Verification items for the finished model (mm, model axes). Coordinates: 2 decimals unless noted, no trailing zeros. Write each loop counter-clockwise with the first axis right and the second up, starting at its lowest first coordinate (ties: lowest second). Pieces come first, ordered by that corner, then holes. Notation, with made-up numbers: (32, 44) -> (61, 44) arc R25 cw to (61, 76) -> close; hole circle Ø11 at (26.25, 60.5). An arc over 180 degrees is marked (long way). Use a Markdown table: item, result. Add a question column.
from build123d import *

# Parameters (mm, degrees)
F1_DEPTH = 10.16


with BuildPart() as f1:
    # F0 (on Top) → F1 (new body)
    with BuildSketch(Plane.XY):
        with BuildLine():
            Line((-127, 50.8), (-127, 0))
            Line((-127, 0), (-115.57, 0))
            ThreePointArc((-115.57, 0), (-107.95, 7.62), (-100.33, 0))
            Line((-100.33, 0), (-88.9, 0))
            ThreePointArc((-88.9, 0), (-81.572297, 35.343604), (-60.79718, 64.860719))
            Line((-60.79718, 64.860719), (-77.096278, 79.650577))
            ThreePointArc((-77.096278, 79.650577), (-87.859909, 79.128047), (-88.382439, 89.891679))
            Line((-88.382439, 89.891679), (-104.681537, 104.681537))
            ThreePointArc((-104.681537, 104.681537), (-121.19962, 79.960478), (-127, 50.8))
        make_face()
        with BuildLine():
            ThreePointArc((-50.8, 127), (-79.960478, 121.19962), (-104.681537, 104.681537))
            Line((-104.681537, 104.681537), (-88.382439, 89.891679))
            ThreePointArc((-88.382439, 89.891679), (-79.994898, 91.879738), (-75.119358, 84.771128))
            ThreePointArc((-75.119358, 84.771128), (-75.630748, 82.026668), (-77.096278, 79.650577))
            Line((-77.096278, 79.650577), (-60.79718, 64.860719))
            ThreePointArc((-60.79718, 64.860719), (-32.688622, 82.672027), (0, 88.9))
            Line((0, 88.9), (0, 100.33))
            ThreePointArc((0, 100.33), (-7.62, 107.95), (0, 115.57))
            Line((0, 115.57), (0, 127))
            Line((0, 127), (-50.8, 127))
        make_face()
        with BuildLine():
            Line((89.270123, 89.048531), (104.681537, 104.681537))
            ThreePointArc((104.681537, 104.681537), (79.960478, 121.19962), (50.8, 127))
            Line((50.8, 127), (0, 127))
            Line((0, 127), (0, 115.57))
            ThreePointArc((0, 115.57), (5.388154, 113.338154), (7.62, 107.95))
            ThreePointArc((7.62, 107.95), (5.388154, 102.561846), (0, 100.33))
            Line((0, 100.33), (0, 88.9))
            ThreePointArc((0, 88.9), (34.215472, 82.051883), (63.159593, 62.562575))
            Line((63.159593, 62.562575), (78.571008, 78.19558))
            ThreePointArc((78.571008, 78.19558), (78.49409, 88.971613), (89.270123, 89.048531))
        make_face()
        with BuildLine():
            Line((115.57, 0), (127, 0))
            Line((127, 0), (127, 50.8))
            ThreePointArc((127, 50.8), (121.19962, 79.960478), (104.681537, 104.681537))
            Line((104.681537, 104.681537), (89.270123, 89.048531))
            ThreePointArc((89.270123, 89.048531), (90.950075, 86.56321), (91.540565, 83.622056))
            ThreePointArc((91.540565, 83.622056), (86.861719, 76.592545), (78.571008, 78.19558))
            Line((78.571008, 78.19558), (63.159593, 62.562575))
            ThreePointArc((63.159593, 62.562575), (82.213435, 33.82545), (88.9, 0))
            Line((88.9, 0), (100.33, 0))
            ThreePointArc((100.33, 0), (107.95, 7.62), (115.57, 0))
        make_face()
        with BuildLine():
            Line((88.958455, -89.357986), (104.681537, -104.681537))
            ThreePointArc((104.681537, -104.681537), (121.19962, -79.960478), (127, -50.8))
            Line((127, -50.8), (127, 0))
            Line((127, 0), (115.57, 0))
            ThreePointArc((115.57, 0), (107.95, -7.62), (100.33, 0))
            Line((100.33, 0), (88.9, 0))
            ThreePointArc((88.9, 0), (81.986502, -34.371843), (62.321292, -63.397685))
            Line((62.321292, -63.397685), (78.044374, -78.721236))
            ThreePointArc((78.044374, -78.721236), (86.372107, -76.981033), (91.121415, -84.039611))
            ThreePointArc((91.121415, -84.039611), (90.559993, -86.910304), (88.958455, -89.357986))
        make_face()
        with BuildLine():
            Line((0, -115.57), (0, -127))
            Line((0, -127), (50.8, -127))
            ThreePointArc((50.8, -127), (79.960478, -121.19962), (104.681537, -104.681537))
            Line((104.681537, -104.681537), (88.958455, -89.357986))
            ThreePointArc((88.958455, -89.357986), (78.18304, -89.496652), (78.044374, -78.721236))
            Line((78.044374, -78.721236), (62.321292, -63.397685))
            ThreePointArc((62.321292, -63.397685), (33.668648, -82.277774), (0, -88.9))
            Line((0, -88.9), (0, -100.33))
            ThreePointArc((0, -100.33), (5.388154, -102.561846), (7.62, -107.95))
            ThreePointArc((7.62, -107.95), (5.388154, -113.338154), (0, -115.57))
        make_face()
        with BuildLine():
            ThreePointArc((-104.681537, -104.681537), (-79.960478, -121.19962), (-50.8, -127))
            Line((-50.8, -127), (0, -127))
            Line((0, -127), (0, -115.57))
            ThreePointArc((0, -115.57), (-7.62, -107.95), (0, -100.33))
            Line((0, -100.33), (0, -88.9))
            ThreePointArc((0, -88.9), (-34.133071, -82.086195), (-63.033834, -62.689279))
            Line((-63.033834, -62.689279), (-78.491774, -78.275104))
            ThreePointArc((-78.491774, -78.275104), (-76.823745, -80.754866), (-76.237686, -83.685408))
            ThreePointArc((-76.237686, -83.685408), (-80.927144, -90.719349), (-89.223597, -89.095712))
            Line((-89.223597, -89.095712), (-104.681537, -104.681537))
        make_face()
        with BuildLine():
            ThreePointArc((-127, -50.8), (-121.19962, -79.960478), (-104.681537, -104.681537))
            Line((-104.681537, -104.681537), (-89.223597, -89.095712))
            ThreePointArc((-89.223597, -89.095712), (-89.26799, -78.319496), (-78.491774, -78.275104))
            Line((-78.491774, -78.275104), (-63.033834, -62.689279))
            ThreePointArc((-63.033834, -62.689279), (-82.179431, -33.907979), (-88.9, 0))
            Line((-88.9, 0), (-100.33, 0))
            ThreePointArc((-100.33, 0), (-107.95, -7.62), (-115.57, 0))
            Line((-115.57, 0), (-127, 0))
            Line((-127, 0), (-127, -50.8))
        make_face()
    extrude(amount=F1_DEPTH)


solid = f1.part
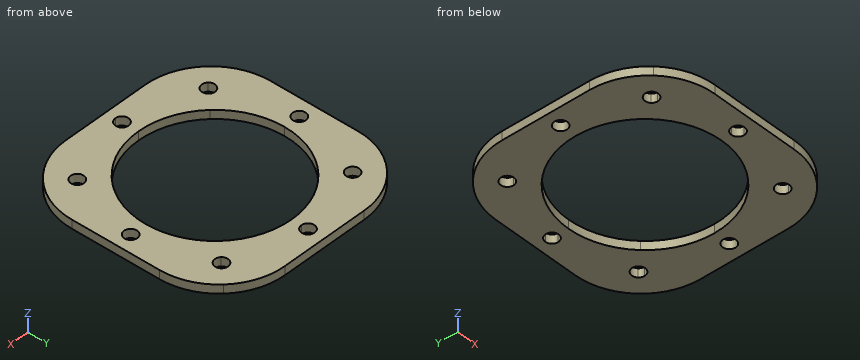
1) Cross-section at B-B on y = 58.5. Record the boundary of the cut face in (x, z).
2) Cross-section at C-C on z = 8. Give the number of separate pieces and of enclosed holes in the cut face, then the cut area to 3 significant figures.
3) Gauge pin test, flat end, axial feed: pin 1 (13.5 mm diameter, centred on x = -107.95, y = 0, fed in from +Z). Record the tip position at first contact, or that the pin passes through.
4) Cross-section at A-A on x = 107.95. Record the boundary of the cut face in (y, z), then the cut area to 3 significant figures.
5) Thickness scan on L1, parallel to Y at x = 107.95, z = 2.5; L2, parallel to X at y = -23.5, z = 4; L3, parallel to Y at x = 3, z = 4.5. Record the ranges inside material, lowest first.
Returned:
| question | item | result |
|---|---|---|
| 1 | outline | (-126.61, 0) -> (-66.94, 0) -> (-66.94, 10.16) -> (-126.61, 10.16) -> close; (66.94, 0) -> (126.61, 0) -> (126.61, 10.16) -> (66.94, 10.16) -> close |
| 2 | separate pieces | 1 |
| 2 | enclosed holes | 9 |
| 2 | area | 33,200 mm² |
| 3 | pin 1 | passes through |
| 4 | outline | (-101.2, 0) -> (-7.62, 0) -> (-7.62, 10.16) -> (-101.2, 10.16) -> close; (7.62, 0) -> (101.2, 0) -> (101.2, 10.16) -> (7.62, 10.16) -> close |
| 4 | area | 1,900 mm² |
| 5 | L1 | y = -101.2 to -7.62, 7.62 to 101.2 |
| 5 | L2 | x = -127 to -85.74, 85.74 to 127 |
| 5 | L3 | y = -127 to -114.95, -100.95 to -88.85, 88.85 to 100.95, 114.95 to 127 |
